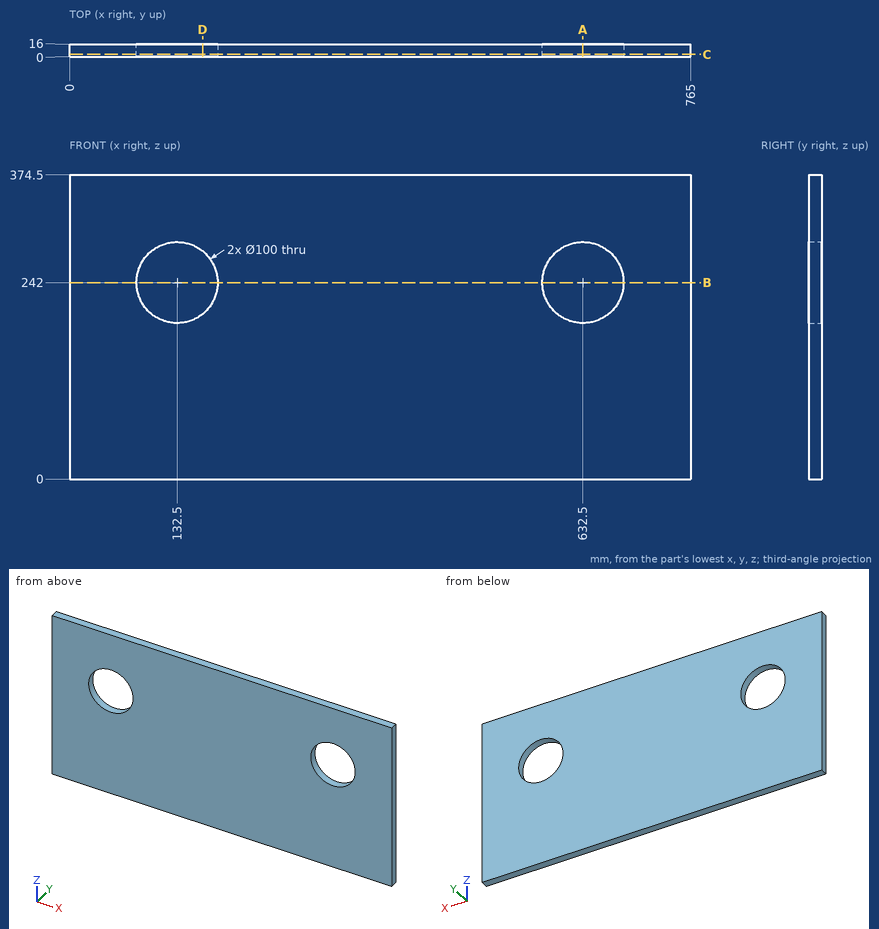
Part print with two shaded views. Sizes in mm from the minimum x, y, z corner. Coordinates: 2 decimals unless noted, no trailing zeros. Write each loop counter-clockwise with the first axis right and the second up, starting at its lowest first coordinate (ties: lowest second). Pieces come first, ordered by that corner, then holes. Notation, with made-up numbers: (14, -6.75) -> (37, -6.75) arc R18 cw to (37, 9.25) -> close; hole circle Ø10 at (88, 56). An arc over 180 degrees is marked (long way). Return JSON: item names as keys, results as strings. Group by question number.
Q1. Cut at B-B, the plane z = 242. Give the cut face in (x, y), then the cut area to 3 significant figures.
Q2. Cut at D-D, the plane x = 164. Give the cut face in (y, z).
Q3. Cut at A-A, the plane x = 632.5. Give the cut face in (y, z), then the cut area to 3 significant figures.
Q4. Drill centre lines: line 1 (X direction, y = 6.5, z = 242); line 2 (Z direction, x = 132.5, y = 4); line 3 (X direction, y = 2, z = 201). Where is each one in solid material? Low to high.
Q5. Cut at C-C, the plane y = 3.25. Give the cut face in (x, z), then the cut area to 3 significant figures.
Returned:
{
 "1": {"outline": "(0, 0) -> (82.5, 0) -> (82.5, 16) -> (0, 16) -> close; (182.5, 0) -> (582.5, 0) -> (582.5, 16) -> (182.5, 16) -> close; (682.5, 0) -> (765, 0) -> (765, 16) -> (682.5, 16) -> close", "area": "9,040 mm2"},
 "2": {"outline": "(0, 0) -> (16, 0) -> (16, 203.17) -> (0, 203.17) -> close; (0, 280.83) -> (16, 280.83) -> (16, 374.5) -> (0, 374.5) -> close"},
 "3": {"outline": "(0, 0) -> (16, 0) -> (16, 192) -> (0, 192) -> close; (0, 292) -> (16, 292) -> (16, 374.5) -> (0, 374.5) -> close", "area": "4,390 mm2"},
 "4": {"line 1": "x = 0 to 82.5, 182.5 to 582.5, 682.5 to 765", "line 2": "z = 0 to 192, 292 to 374.5", "line 3": "x = 0 to 103.88, 161.12 to 603.88, 661.12 to 765"},
 "5": {"outline": "(0, 0) -> (765, 0) -> (765, 374.5) -> (0, 374.5) -> close; hole circle Ø100 at (132.5, 242); hole circle Ø100 at (632.5, 242)", "area": "271,000 mm2"}
}
